from build123d import *

# Parameters (mm, degrees)
SKETCH1_W               = 7.250077802
SKETCH1_H               = 2.953476685
CUT_EXTRUDE1_DEPTH      = 20.334926531
CUT_EXTRUDE1_DEPTH_BACK = 20.334926531
SKETCH2_R               = 1.190625


with BuildPart() as part:
    # Sketch1 → Revolve1 (revolve)
    with BuildSketch(Plane.XY, mode=Mode.PRIVATE) as revolve1_sk:
        with Locations((-3.625038901, 3.064238343)):
            Rectangle(SKETCH1_W, SKETCH1_H)
        Polygon((-14.689288069, 1.5875), (-7.250077802, 1.5875), (-7.250077802, 4.540976685), (-7.250077802, 8.89), (-14.689288069, 8.89), align=None)
    revolve(revolve1_sk.sketch.rotate(Axis((0, 0, 0), (-1, 0, 0)), 90), axis=Axis((0, 0, 0), (-1, 0, 0)))

    # Sketch2 → Cut-Extrude1 (cut, two sides: drawn at the far end of the back side and taken through both)
    with BuildSketch(Plane(origin=(0, 0, 0), x_dir=(1, 0, 0), z_dir=(0, 1, 0)).offset(-CUT_EXTRUDE1_DEPTH_BACK)):
        with Locations(Location((-3.529556327, 0, 0), (0, 0, 270))):
            Circle(SKETCH2_R)
    extrude(amount=CUT_EXTRUDE1_DEPTH + CUT_EXTRUDE1_DEPTH_BACK, mode=Mode.SUBTRACT)


solid = part.part
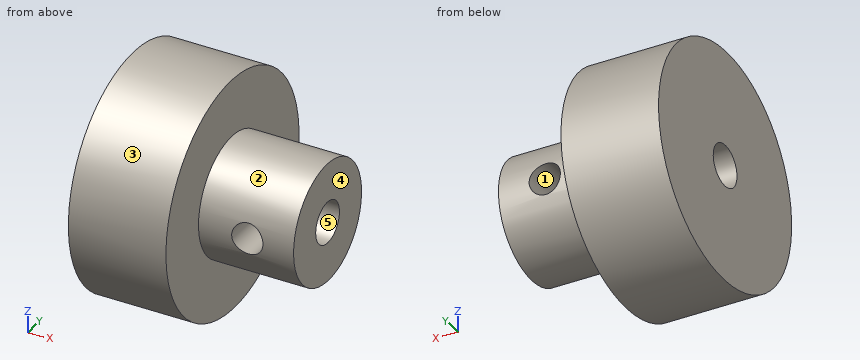
Can you work these out from the model? Positions are in its coordinate system, mm. Face numbers are marked on the shaded views. A direction names the side the tool comes from. Coordinates: 2 decimals unless noted, no trailing zeros. Write each loop counter-clockwise with the first axis right and the second up, starting at its lowest first coordinate (ties: lowest second). Pieces come first, ordered by that corner, then holes.
Q1. Which directions (+Z, -Z, +X, -X, +Y, -Y) give clear straight access to the entire face, cutting with the end or side of a thin tool? Please do the marked faces 1 and 2.
Results found:
face 1: +Y, -Y
face 2: +X
Q2. Imagine slicing it at B-B, the plane z = 0. List the corners of the cut face in (x, y) for me.
Results found:
outline: (-14.69, -8.89) - (-7.25, -8.89) - (-7.25, -4.54) - (-4.72, -4.54) - (-4.72, -1.59) - (-14.69, -1.59) - close; (-14.69, 1.59) - (-4.72, 1.59) - (-4.72, 4.54) - (-7.25, 4.54) - (-7.25, 8.89) - (-14.69, 8.89) - close; (-2.34, -4.54) - (0, -4.54) - (0, -1.59) - (-2.34, -1.59) - close; (-2.34, 1.59) - (0, 1.59) - (0, 4.54) - (-2.34, 4.54) - close
Q3. If we mould it in two halves opening along Z, with no side actions, what happens to the marked faces 3, 4 and 5? For each: +Z half, -Z half, draft (parallel to the pull), parting line (faces both ways), or undercut.
Results found:
face 3: parting line
face 4: draft
face 5: undercut
Q4. Imagine slicing it at D-D, the plane z = -7.5. List the corners of the cut face in (x, y) for me, plus the area to 3 significant figures.
Results found:
outline: (-14.69, -4.77) - (-7.25, -4.77) - (-7.25, 4.77) - (-14.69, 4.77) - close
area: 71.0 mm2
Q5. Please list where these lines run through material, in increasing order: L1, parallel to X at y = -2.35, z = 0; L2, parallel to Y at x = -8, z = 0; L3, parallel to Y at x = -5, z = -0.5.
Results found:
L1: x = -14.69 to -4.72, -2.34 to 0
L2: y = -8.89 to -1.59, 1.59 to 8.89
L3: y = -4.51 to -1.51, 1.51 to 4.51
Q6. Imagine slicing it at C-C, the plane x = -1.25. List the corners of the cut face in (y, z) for me (1 decimal), plus the area to 3 significant figures.
Results found:
outline: circle Ø9.1 at (0, 0); hole circle Ø3.2 at (0, 0)
area: 56.9 mm2
Q7. Imagine slicing it at A-A, the plane y = 0. List the corners of the cut face in (x, z) for me, plus the area to 3 significant figures.
Results found:
outline: (-14.69, -8.89) - (-7.25, -8.89) - (-7.25, -4.54) - (0, -4.54) - (0, -1.59) - (-14.69, -1.59) - close; (-14.69, 1.59) - (0, 1.59) - (0, 4.54) - (-7.25, 4.54) - (-7.25, 8.89) - (-14.69, 8.89) - close
area: 151 mm2
Q8. For P1, Ø3, axis at x = -3.53, z = 0, coming from the -Y side; P2, Ø6, axis at x = -9, y = 6.5, coming from the +Z side; P3, Ø5, axis at x = -6, z = -6, coming from the +Y side, each with a flat end and sliding along its axis, tell me the tip position at first contact or that it passes through.
Results found:
P1: stops at y = -4.54
P2: stops at z = 8.17
P3: stops at y = 8.02
